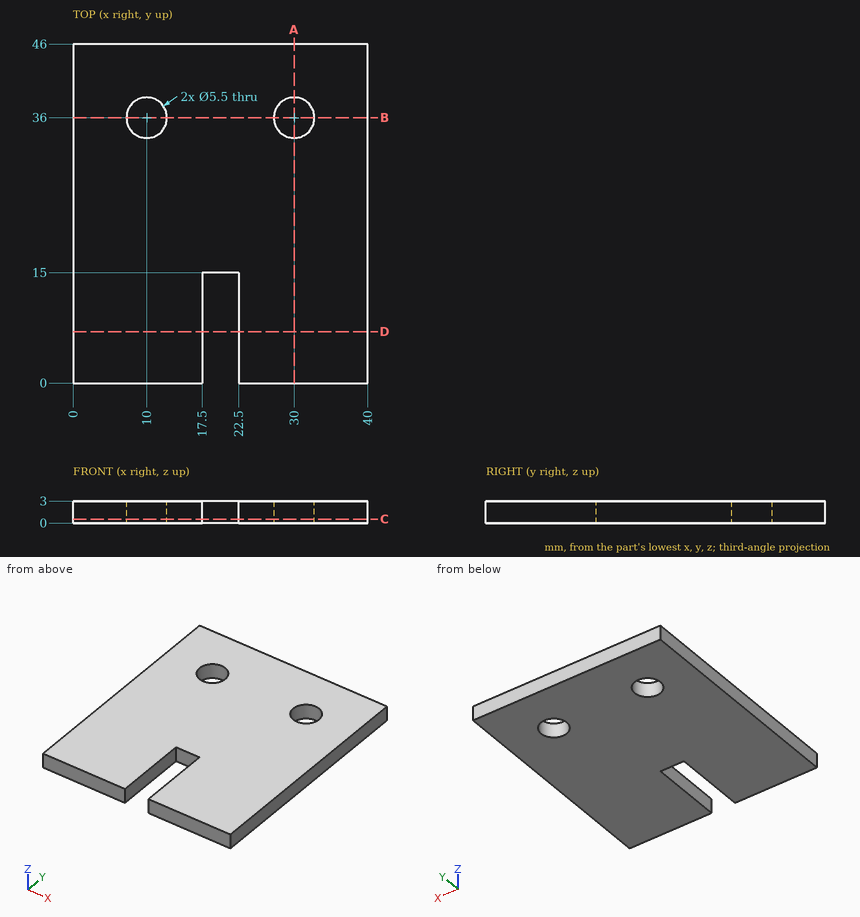
Job drawing, mm, ordinate dimensions from the low corner. One solid piece. Round coordinates to 2 decimals unless told otherwise and drop trailing zeros. Order: outer loops, then holes, each group sorted by start corner. A loop starts at its lowest first (then second) coordinate and runs counter-clockwise, first axis right, second up. Notation, with made-up numbers: (36.5, 11.25) -> (71.5, 11.25) arc R21 cw to (71.5, 45.25) -> close; hole circle Ø3 at (-7.5, 88). An arc over 180 degrees is marked (long way). Answer in a Markdown table with one row per item.
1) Wall check: L1, parallel to Y at x = 10, z = 1.2; L2, parallel to X at y = 13, z = 0.15; L3, parallel to Y at x = 28, z = 1.1. Give the ranges that are in metal, low to high.
Values:
| item | result |
|---|---|
| L1 | 0 to 33.25, 38.75 to 46 |
| L2 | 0 to 17.5, 22.5 to 40 |
| L3 | 0 to 34.11, 37.89 to 46 |
2) Band-saw the part on B-B on y = 36. Give the cut face in (x, z).
Values:
| item | result |
|---|---|
| outline | (0, 0) -> (7.25, 0) -> (7.25, 3) -> (0, 3) -> close; (12.75, 0) -> (27.25, 0) -> (27.25, 3) -> (12.75, 3) -> close; (32.75, 0) -> (40, 0) -> (40, 3) -> (32.75, 3) -> close |
3) Band-saw the part on D-D on y = 7. Give the cut face in (x, z).
Values:
| item | result |
|---|---|
| outline | (0, 0) -> (17.5, 0) -> (17.5, 3) -> (0, 3) -> close; (22.5, 0) -> (40, 0) -> (40, 3) -> (22.5, 3) -> close |
4) Pin check, flat tip, straight feed: P1, Ø1.5, axis at x = 20, z = 1.5, coming from the -Y side. Stop position of the tip, or through.
Values:
| item | result |
|---|---|
| P1 | y = 15 |
5) Band-saw the part on C-C on z = 0.55. Give the cut face in (x, y), and give its area (3 significant figures).
Values:
| item | result |
|---|---|
| outline | (0, 0) -> (17.5, 0) -> (17.5, 15) -> (22.5, 15) -> (22.5, 0) -> (40, 0) -> (40, 46) -> (0, 46) -> close; hole circle Ø5.5 at (10, 36); hole circle Ø5.5 at (30, 36) |
| area | 1,720 mm2 |
6) Band-saw the part on A-A on x = 30. Give the cut face in (y, z), and give its area (4 significant figures).
Values:
| item | result |
|---|---|
| outline | (0, 0) -> (33.25, 0) -> (33.25, 3) -> (0, 3) -> close; (38.75, 0) -> (46, 0) -> (46, 3) -> (38.75, 3) -> close |
| area | 121.5 mm2 |
